Check sheet for the modelled part. Datum: model origin and axes. Units: mm. Face numbers are marked on the shaded views. A direction names the side the tool comes from. Coordinates: 2 decimals unless noted, no trailing zeros. Order: outer loops, then holes, each group sorted by start corner. A loop starts at its lowest first (then second) coordinate and runs counter-clockwise, first axis right, second up.
1. Set-up check for the marked faces 5 and 6: record each of +Z, -Z, +X, -X, +Y, -Y from which the full face is reachable in a straight line by a thin tool's end or side.
2. Cross-section at A-A (z = 22). Enter the section's corners in (x, y), then the cut area to 3 significant figures.
3. Draft check along Z on the marked faces 1, 2, 3 and 4. Enter one of: released by +Z, released by -Z, zero draft, split by the parting line, or undercut.
4. Thickness scan on line 1 (Z direction, x = 38, y = 0.8); line 2 (Y direction, x = 15, z = 22). Record the ranges inside material, lowest first.
```python
from build123d import *

# Parameters (mm, degrees)
SKETCH_1_W          = 150
SKETCH_1_H          = 80
EXTRUDE_1_DEPTH     = 45
SKETCH_2_R          = 32.5
SKETCH_2_R_2        = 20.5
CUT_EXTRUDE_1_DEPTH = 1.5


with BuildPart() as part:
    # 草图1 → 凸台-拉伸1 (new body)
    with BuildSketch(Plane(origin=(0, 0, 0), x_dir=(1, 0, 0), z_dir=(0, 1, 0))):
        Rectangle(SKETCH_1_W, SKETCH_1_H)
    extrude(amount=EXTRUDE_1_DEPTH)

    # 草图2 → 切除-拉伸1 (cut)
    with BuildSketch(Plane.XZ):
        with Locations((38, 0)):
            Circle(SKETCH_2_R)
        with Locations((38, 0)):
            Circle(SKETCH_2_R_2, mode=Mode.SUBTRACT)
        with Locations((-38, 0)):
            Circle(SKETCH_2_R)
        with Locations((-38, 0)):
            Circle(SKETCH_2_R_2, mode=Mode.SUBTRACT)
    extrude(amount=-CUT_EXTRUDE_1_DEPTH, mode=Mode.SUBTRACT)


solid = part.part
```
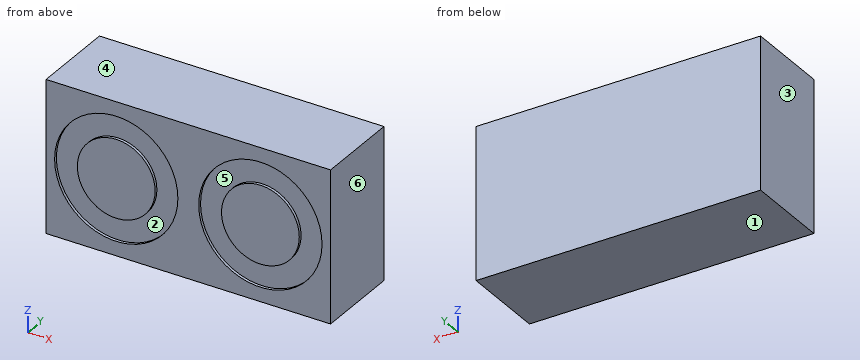
Data:
1. face 5: -Y
1. face 6: +Z, -Z, +X, +Y, -Y
2. outline: (-75, 0) - (-61.92, 0) - (-61.92, 1.5) - (-14.08, 1.5) - (-14.08, 0) - (14.08, 0) - (14.08, 1.5) - (61.92, 1.5) - (61.92, 0) - (75, 0) - (75, 45) - (-75, 45) - close
2. area: 6,610 mm2
3. face 1: released by -Z
3. face 2: undercut
3. face 3: zero draft
3. face 4: released by +Z
4. line 1: z = -40 to -32.5, -20.5 to 20.5, 32.5 to 40
4. line 2: y = 1.5 to 45
